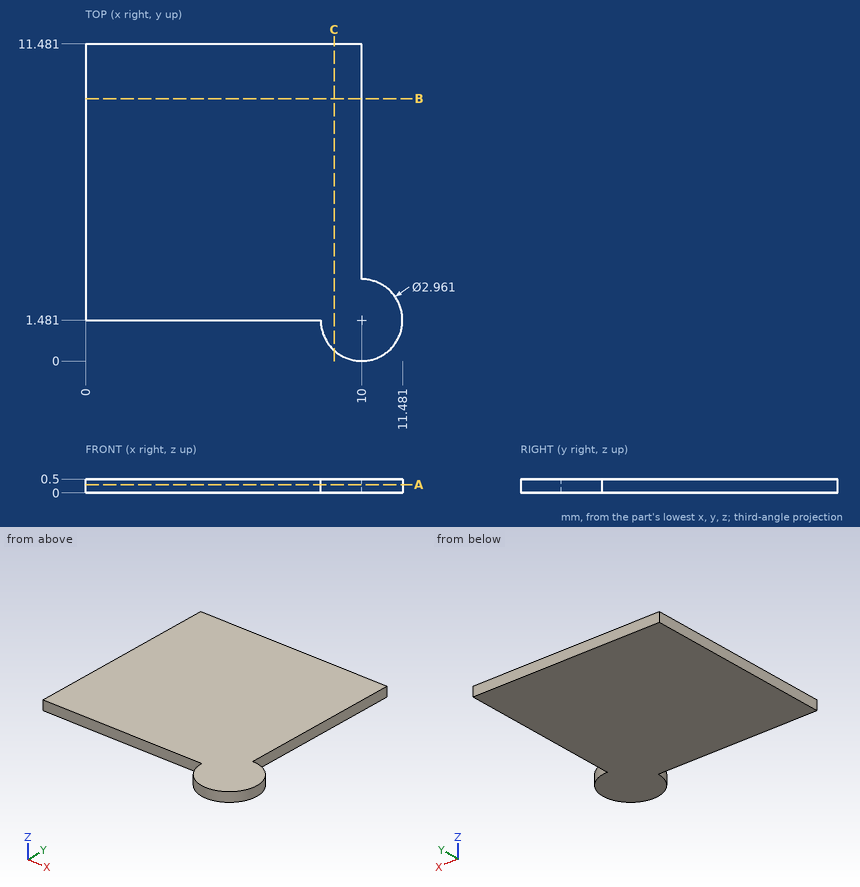
Answer from the drawing. Dimensions are ordinates in mm from the lowest x, y and z of the part. Give positions to 0.01 mm unless a question says otherwise; leave off trailing zeros. Write each loop counter-clockwise with the first axis right and the second up, starting at its lowest first coordinate (ties: lowest second). Pieces come first, ordered by that corner, then holes. Notation, with made-up numbers: (73, 15.25) - (124, 15.25) arc R22 cw to (124, 32.25) - close; hole circle Ø11 at (42.5, 31.25). An arc over 180 degrees is marked (long way). Answer in a Markdown table with one row per item. Add a question column.
Item 1: Section A-A, the plane z = 0.3 is taken. Write down the section's boundary in (x, y).
Item 2: Find the intervals of material crossed by L1, parallel to Y at x = 6.75, z = 0.15; L2, parallel to X at y = 4.5, z = 0.25; L3, parallel to X at y = 1.25, z = 0.2, in increasing order.
Item 3: Section C-C, the plane x = 9 is taken. Write down the section's boundary in (y, z).
Item 4: Section B-B, the plane y = 9.5 is taken. Write down the section's boundary in (x, z).
Recorded:
| question | item | result |
|---|---|---|
| 1 | outline | (0, 1.48) - (8.52, 1.48) arc R1.48 ccw (long way) to (10, 2.96) - (10, 11.48) - (0, 11.48) - close |
| 2 | L1 | y = 1.48 to 11.48 |
| 2 | L2 | x = 0 to 10 |
| 2 | L3 | x = 8.54 to 11.46 |
| 3 | outline | (0.39, 0) - (11.48, 0) - (11.48, 0.5) - (0.39, 0.5) - close |
| 4 | outline | (0, 0) - (10, 0) - (10, 0.5) - (0, 0.5) - close |
